CAD build for the part. Positions are in the model's coordinates, mm. A direction names the side the tool comes from. Round coordinates to 2 decimals unless told otherwise and drop trailing zeros. Order: outer loops, then holes, each group sorted by start corner. A loop starts at its lowest first (then second) coordinate and runs counter-clockwise, first axis right, second up. Notation, with made-up numbers: (24, 59) -> (33, 59) arc R22 cw to (33, 94) -> close; hole circle Ø2 at (-10.75, -3). An arc over 180 degrees is marked (long way). Answer as CSV lines item,"result". Start each with the question number.
from build123d import *

# Parameters (mm, degrees)
BOSS_EXTRUDE1_DEPTH = 12.7
SKETCH3_W           = 4.233333333
SKETCH3_H           = 15.24
CUT_EXTRUDE1_DEPTH  = 20.32
FILLET1_R           = 2.54
FILLET2_R           = 2.54
SCALE1_SCALE        = 3


with BuildPart() as part:
    # Sketch1 → Boss-Extrude1 (new body)
    with BuildSketch(Plane.XY):
        Polygon((0, 0), (0, 25.4), (5.08, 25.4), (5.08, 20.32), (20.32, 5.08), (25.4, 5.08), (25.4, 0), align=None)
    extrude(amount=BOSS_EXTRUDE1_DEPTH)

    # Sketch3 → Cut-Extrude1 (cut)
    with BuildSketch(Plane(origin=(25.4, 0, 0), x_dir=(0, 0, -1), z_dir=(1, 0, 0))):
        with Locations((-10.583333334, 12.7)):
            Rectangle(SKETCH3_W, SKETCH3_H)
        with Locations((-2.116666667, 12.7)):
            Rectangle(SKETCH3_W, SKETCH3_H)
    extrude(amount=-CUT_EXTRUDE1_DEPTH, mode=Mode.SUBTRACT)

    # Fillet1
    fillet1_edges = [part.edges().sort_by_distance(p)[0] for p in [
        (5.08, 5.08, 10.583333333),
        (5.08, 5.08, 2.116666667),
    ]]
    fillet(fillet1_edges, radius=FILLET1_R)

    # Fillet2
    fillet2_edges = [part.edges().sort_by_distance(p)[0] for p in [
        (5.08, 20.32, 6.35),
        (20.32, 5.08, 6.35),
    ]]
    fillet(fillet2_edges, radius=FILLET2_R)


with BuildPart() as part_1:
    # Scale1: scaled about (8.45857593, 8.45857593, 6.35)
    add(part.part.scale(SCALE1_SCALE).moved(Location((-16.91715186, -16.91715186, -12.7))))


solid = part_1.part
Item 1: Pin check, flat tips, straight feed: pin 1 (12 mm diameter, centred on x = 34.5, z = 18, fed in from +Y); pin 2 (4 mm diameter, centred on x = 10, y = 1.5, fed in from -Z); pin 3 (2 mm diameter, centred on x = 0, z = 5, fed in from +Y). Stop position of each tip, or through.
Item 2: Tool access for faces 1 (the flat face through (-1.677, 33, 15)), 2 (the cylindrical face through (0.5, 0.61, -6.44)), 3 (the flat face through (12, 12, 12.7)): list every direction of +Z, -Z, +X, -X, +Y, -Y with a clear straight run to the whole face (end or side of a thin tool).
Item 3: Probe line 1 (X direction, y = 52, z = -11); line 2 (Z direction, x = 13.5, y = 11.5). List the from-to ranges inside material, lowest first.
Item 4: Band-saw the part on D-D, the plane z = -1. Give the cut face in (x, y).
Item 5: Band-saw the part on C-C, the plane y = 13. Give the cut face in (x, z).
Item 6: Band-saw the part on B-B, the plane x = 32. Give the cut face in (y, z), and give its area (3 significant figures).
Item 7: Band-saw the part on A-A, the plane z = 5. Give the cut face in (x, y), and give its area (3 significant figures).
Values:
1,pin 1,"y = 10.68"
1,pin 2,"z = 0"
1,pin 3,"y = 44.06"
2,face 1,"+X, +Y"
2,face 2,"-Z, +X, +Y"
2,face 3,"+Z, +X, +Y"
3,line 1,"-16.92 to -1.68"
3,line 2,"0 to 12.7"
4,outline,"(-16.92, -16.92) -> (59.28, -16.92) -> (59.28, -1.68) -> (5.94, -1.68) arc R7.62 cw to (-1.68, 5.94) -> (-1.68, 59.28) -> (-16.92, 59.28) -> close"
5,outline,"(-16.92, -12.7) -> (-1.68, -12.7) -> (-1.68, 0) -> (29.37, 0) -> (29.37, 12.7) -> (-1.68, 12.7) -> (-1.68, 25.4) -> (-16.92, 25.4) -> close"
6,outline,"(-16.92, -12.7) -> (-1.68, -12.7) -> (-1.68, 0) -> (10.37, 0) -> (10.37, 12.7) -> (-1.68, 12.7) -> (-1.68, 25.4) -> (-16.92, 25.4) -> close"
6,area,"734 mm²"
7,outline,"(-16.92, -16.92) -> (59.28, -16.92) -> (59.28, -1.68) -> (47.2, -1.68) arc R7.62 cw to (41.81, 0.55) -> (0.55, 41.81) arc R7.62 cw to (-1.68, 47.2) -> (-1.68, 59.28) -> (-16.92, 59.28) -> close"
7,area,"3,140 mm²"
